Here's how the part is built. I have some questions about the finished solid (model axes, mm). A direction names the side the tool comes from. Round coordinates to 2 decimals unless told otherwise and drop trailing zeros. Loops run counter-clockwise (first coordinate to the right, second up) from the corner with the lowest first, then second, coordinate; pieces in that order, holes last. Notation, with made-up numbers: M 87,10 L 146,10 A11 cw 146,18 Z; hole C 58,-35 d1. An arc over 180 degrees is marked long. Answer as a JSON object with one key per item and string values.
from build123d import *

# Parameters (mm, degrees)
SKETCH1_R           = 85
BOSS_EXTRUDE1_DEPTH = 130
SKETCH2_R           = 26
CUT_EXTRUDE1_DEPTH  = 124
SKETCH3_R           = 75
SKETCH3_R_2         = 70
BOSS_EXTRUDE2_DEPTH = 72.35


with BuildPart() as part:
    # Sketch1 → Boss-Extrude1 (new body)
    with BuildSketch(Plane(origin=(0, 0, 0), x_dir=(1, 0, 0), z_dir=(0, 1, 0))):
        Circle(SKETCH1_R)
    extrude(amount=BOSS_EXTRUDE1_DEPTH)

    # Sketch2 → Cut-Extrude1 (cut)
    with BuildSketch(Plane(origin=(0, 130, 0), x_dir=(1, 0, 0), z_dir=(0, 1, 0))):
        Circle(SKETCH2_R)
    extrude(amount=-CUT_EXTRUDE1_DEPTH, mode=Mode.SUBTRACT)

    # Sketch3 → Boss-Extrude2 (add)
    with BuildSketch(Plane(origin=(0, 130, 0), x_dir=(1, 0, 0), z_dir=(0, 1, 0))):
        Circle(SKETCH3_R)
        Circle(SKETCH3_R_2, mode=Mode.SUBTRACT)
    extrude(amount=BOSS_EXTRUDE2_DEPTH)


solid = part.part
Item 1: I want a section at A-A, the plane x = 0. Please give me the cut outline in (y, z).
Resolved:
{"outline": "M 0,-85 L 130,-85 L 130,-75 L 202.35,-75 L 202.35,-70 L 130,-70 L 130,-26 L 6,-26 L 6,26 L 130,26 L 130,70 L 202.35,70 L 202.35,75 L 130,75 L 130,85 L 0,85 Z"}
Item 2: I want a section at B-B, the plane z = 0. Please give me the cut outline in (x, y), then the cut area to 3 significant figures.
Resolved:
{"outline": "M -85,0 L 85,0 L 85,130 L 75,130 L 75,202.35 L 70,202.35 L 70,130 L 26,130 L 26,6 L -26,6 L -26,130 L -70,130 L -70,202.35 L -75,202.35 L -75,130 L -85,130 Z", "area": "16,400 mm²"}
Item 3: Please list where these lines run through material, in increasing order: probe 1 along Z at (x, y) = (0, 170.5); probe 2 along X at (y, z) = (33, 0). Write a range as from..to.
Resolved:
{"probe 1": "-75..-70, 70..75", "probe 2": "-85..-26, 26..85"}
Item 4: I want a section at C-C, the plane y = 167.5. Please give me the cut outline in (x, z), then the cut area to 3 significant figures.
Resolved:
{"outline": "C 0,0 d150; hole C 0,0 d140", "area": "2,280 mm²"}
Item 5: On a 3-axis mill with a long thin cutter (end or side, diameter ignored), from which of +Z, -Z, +X, -X, +Y, -Y can I reach the whole of each face in a straight line? I mean faces 1 (the face through (-55.55, 165.669, 42.594)), 2 (the face through (-1, 0, -1)). Say none if no direction works.
Resolved:
{"face 1": "+Y", "face 2": "+Z, -Z, +X, -X, -Y"}
Item 6: I'm going to push flat-ended pins straight in: pin 1 Ø5 at (y, z) = (23.5, -41) entering from +X; pin 2 Ø12 at (x, y) = (-18.5, 128.5) entering from -Z; pin 3 Ø5 at (x, z) = (-59, 61.5) entering from +Y. Where does each tip first touch, or does it pass through?
Resolved:
{"pin 1": "x = 75.78", "pin 2": "z = -84.08", "pin 3": "y = 130"}
Item 7: I want a section at D-D, the plane y = 35. Please give me the cut outline in (x, z), then the cut area to 3 significant figures.
Resolved:
{"outline": "C 0,0 d170; hole C 0,0 d52", "area": "20,600 mm²"}
